Check sheet for the drawn part. Datum: minimum x, y, z corner. Units: mm. A direction names the side the tool comes from. Round coordinates to 2 decimals unless told otherwise and drop trailing zeros. Loops run counter-clockwise (first coordinate to the right, second up) from the corner with the lowest first, then second, coordinate; pieces in that order, holes last.
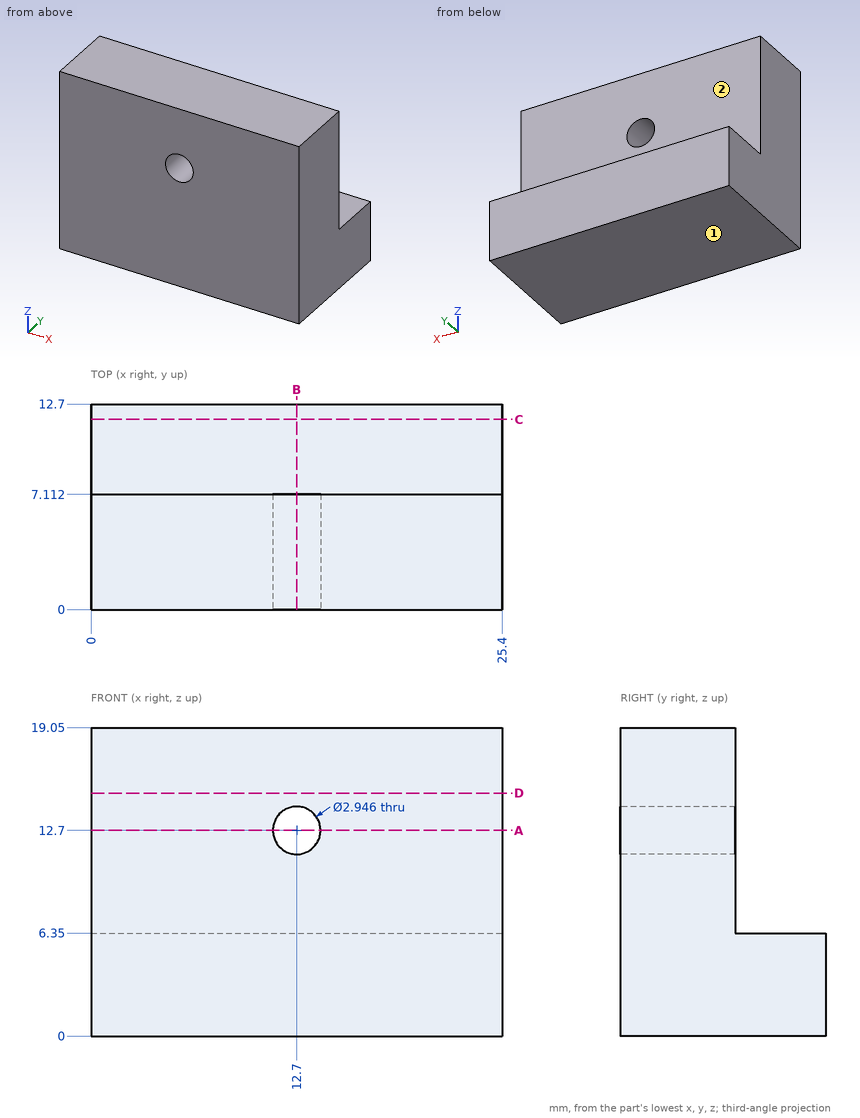
1) Gauge pin test, flat ends, axial feed: pin 1 (1.7 mm diameter, centred on x = 13.5, y = 10.5, fed in from +Z); pin 2 (1.8 mm diameter, centred on x = 12.7, z = 12.7, fed in from -Y). Record the tip position at first contact, or that the pin passes through.
Report:
pin 1: stops at z = 6.35
pin 2: passes through
2) Sectioned sample at D-D, the plane z = 15. Record the cut outline in (x, y), then the cut area to 3 significant figures.
Report:
outline: (0, 0) - (25.4, 0) - (25.4, 7.11) - (0, 7.11) - close
area: 181 mm2
3) Access from +Z, -Z, +X, -X, +Y, -Y to the whole of each face (thin tool, end or side, straight path). Record for the marked faces 1 and 2.
Report:
face 1: -Z, +X, -X, +Y, -Y
face 2: +Z, +X, -X, +Y
4) Sectioned sample at B-B, the plane x = 12.7. Record the cut outline in (y, z).
Report:
outline: (0, 0) - (12.7, 0) - (12.7, 6.35) - (7.11, 6.35) - (7.11, 11.23) - (0, 11.23) - close; (0, 14.17) - (7.11, 14.17) - (7.11, 19.05) - (0, 19.05) - close
5) Sectioned sample at A-A, the plane z = 12.7. Record the cut outline in (x, y).
Report:
outline: (0, 0) - (11.23, 0) - (11.23, 7.11) - (0, 7.11) - close; (14.17, 0) - (25.4, 0) - (25.4, 7.11) - (14.17, 7.11) - close
6) Scan lines: line 1 along Z through (x, y) = (12.7, 3.5); line 2 along X through (y, z) = (3.25, 12.75); line 3 along Y through (x, z) = (21, 13). Record each from-to range of solid material in increasing order.
Report:
line 1: z = 0 to 11.23, 14.17 to 19.05
line 2: x = 0 to 11.23, 14.17 to 25.4
line 3: y = 0 to 7.11
7) Sectioned sample at C-C, the plane y = 11.75. Record the cut outline in (x, z), then the cut area to 3 significant figures.
Report:
outline: (0, 0) - (25.4, 0) - (25.4, 6.35) - (0, 6.35) - close
area: 161 mm2
